Source: CAD feature listing. Evaluate the final solid. Frame: model axes, mm. Face numbers are marked on the shaded views. A direction names the side the tool comes from. Coordinates: 2 decimals unless noted, no trailing zeros. Order: outer loops, then holes, each group sorted by start corner. A loop starts at its lowest first (then second) coordinate and runs counter-clockwise, first axis right, second up. Notation, with made-up numbers: (44.25, -19.5) - (72.25, -19.5) arc R34 ccw to (72.25, 10.5) - close; hole circle Ø5 at (41.25, -16.75). An arc over 180 degrees is marked (long way). One line per question, with ' | ' between items.
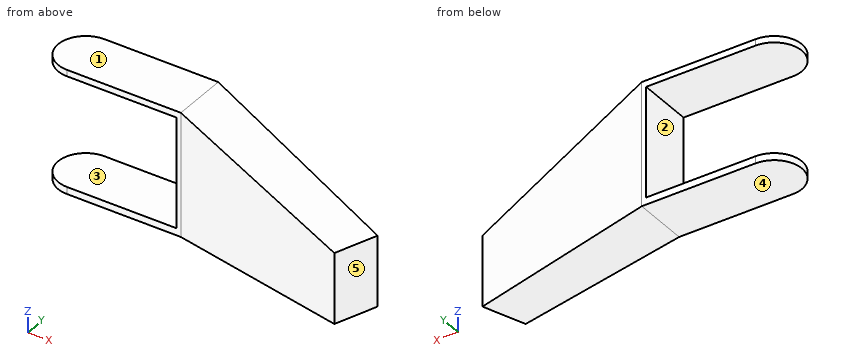
from build123d import *

# Parameters (mm, degrees)
EXTRUDE_1_DEPTH          = 28
CUT_EXTRUDE_1_DEPTH      = 25.1
CUT_EXTRUDE_1_DEPTH_BACK = 24.8
SKETCH_3_W               = 56
SKETCH_3_H               = 25
SKETCH_6_W               = 32
SKETCH_6_H               = 20


with BuildPart() as part:
    # Эскиз1 → Бобышка-Вытянуть1 (new body, symmetric)
    with BuildSketch(Plane.XY):
        with BuildLine():
            Line((0, 12.5), (51.5, 12.5))
            Line((51.5, 12.5), (51.5, -12.5))
            Line((51.5, -12.5), (0, -12.5))
            ThreePointArc((0, -12.5), (-12.5, 0), (0, 12.5))
        make_face()
    extrude(amount=EXTRUDE_1_DEPTH, both=True)

    # Эскиз2 → Вырез-Вытянуть1 (cut, two sides)
    with BuildSketch(Plane.XY) as cut_extrude_1_sk:
        with BuildLine():
            Line((0, 12.5), (49.5, 12.5))
            Line((49.5, 12.5), (49.5, -12.5))
            Line((49.5, -12.5), (0, -12.5))
            ThreePointArc((0, -12.5), (-12.5, 0), (0, 12.5))
        make_face()
    extrude(amount=CUT_EXTRUDE_1_DEPTH, mode=Mode.SUBTRACT)
    extrude(cut_extrude_1_sk.sketch, amount=-CUT_EXTRUDE_1_DEPTH_BACK, mode=Mode.SUBTRACT)

    # Эскиз3 → По сечениям1 section 0
    with BuildSketch(Plane(origin=(51.5, 0, 0), x_dir=(0, 0, -1), z_dir=(1, 0, 0))):
        Rectangle(SKETCH_3_W, SKETCH_3_H)
    # Эскиз6 → По сечениям1 section 1
    with BuildSketch(Plane(origin=(145.469262079, -34.202014333, 0), x_dir=(0, 0, -1), z_dir=(0.939692621, -0.342020143, 0))):
        Rectangle(SKETCH_6_W, SKETCH_6_H)
    loft()


solid = part.part
(1) Set-up query: the marked faces 1 and 2. Return all of +Z, -Z, +X, -X, +Y, -Y with unobstructed straight access to the full face (end or side cutting, diameter ignored); none if empty.
Taken from the geometry:
face 1: +Z, +X, -X, +Y, -Y | face 2: -X, +Y, -Y
(2) Material intervals for L1, parallel to Z at x = 34.5, y = -10; L2, parallel to Y at x = 119, z = 13; L3, parallel to Y at x = 91, z = 6.5, sorted ascending. Write a range as from..to.
Taken from the geometry:
L1: z = -28..-24.8, 25.1..28 | L2: y = -35.68..-13.36 | L3: y = -26.07..-2.63
(3) Cut plane A-A (x = 16.5). Return the cut outline in (y, z).
Taken from the geometry:
outline: (-12.5, -28) - (12.5, -28) - (12.5, -24.8) - (-12.5, -24.8) - close; (-12.5, 25.1) - (12.5, 25.1) - (12.5, 28) - (-12.5, 28) - close
(4) Pull-direction query (Z, two-part tool) for the marked faces 3, 4 and 5; classes: pulls with the +Z half, pulls with the -Z half, needs draft (parallel to the pull), parting line crosses it, or undercut.
Taken from the geometry:
face 3: undercut | face 4: pulls with the -Z half | face 5: needs draft
